Design review of the part built by this model. Coordinates are the model's own, in mm. A direction names the side the tool comes from. Give positions to 0.01 mm unless a question says otherwise; leave off trailing zeros. Write each loop counter-clockwise with the first axis right and the second up, starting at its lowest first coordinate (ties: lowest second). Pieces come first, ordered by that corner, then holes. Notation, with made-up numbers: (32.25, -19) -> (87.25, -19) arc R25 cw to (87.25, 17) -> close; hole circle Ø10 at (-10, -8). An arc over 180 degrees is marked (long way). Use CSV: the item, a comma, the result in double quotes.
```python
from build123d import *

# Parameters (mm, degrees)
SKETCH_1_R      = 7
SKETCH_1_R_2    = 6
EXTRUDE_1_DEPTH = 1
SKETCH_1_4_R    = 6
SKETCH_1_4_R_2  = 5
EXTRUDE_2_DEPTH = 1.5
SKETCH_1_5_R    = 5
SKETCH_1_5_R_2  = 4.25
EXTRUDE_3_DEPTH = 12
EXTRUDE_START   = 5
SKETCH_1_6_R    = 4.25
SKETCH_1_6_W    = 5.5
SKETCH_1_6_H    = 5.5
EXTRUDE_4_DEPTH = 7
SKETCH_1_7_R    = 7
SKETCH_1_7_R_2  = 6
SKETCH_1_7_R_3  = 5
SKETCH_1_7_R_4  = 4.25
SKETCH_1_7_W    = 5.5
SKETCH_1_7_H    = 5.5
SKETCH_1_7_R_5  = 2.1
EXTRUDE_5_DEPTH = 6
FILLET_1_R      = 1
CHAMFER_1_SIZE  = 0.2
CHAMFER_2_SIZE  = 0.3
CHAMFER_3_SIZE  = 0.3


with BuildPart() as part:
    # Sketch 1 → Extrude 1 (new body)
    with BuildSketch(Plane(origin=(0, 0, 0), x_dir=(1, 0, 0), z_dir=(0, 1, 0))):
        with Locations(Location((0, 0, 0), (0, 0, 270))):
            Circle(SKETCH_1_R)
        with Locations(Location((0, 0, 0), (0, 0, 270))):
            Circle(SKETCH_1_R_2, mode=Mode.SUBTRACT)
    extrude(amount=EXTRUDE_1_DEPTH)

    # Sketch 1_4 → Extrude 2 (add)
    with BuildSketch(Plane(origin=(0, 0, 0), x_dir=(1, 0, 0), z_dir=(0, 1, 0))):
        with Locations(Location((0, 0, 0), (0, 0, 270))):
            Circle(SKETCH_1_4_R)
        with Locations(Location((0, 0, 0), (0, 0, 270))):
            Circle(SKETCH_1_4_R_2, mode=Mode.SUBTRACT)
    extrude(amount=EXTRUDE_2_DEPTH)

    # Sketch 1_5 → Extrude 3 (add)
    with BuildSketch(Plane(origin=(0, 0, 0), x_dir=(1, 0, 0), z_dir=(0, 1, 0))):
        with Locations(Location((0, 0, 0), (0, 0, 270))):
            Circle(SKETCH_1_5_R)
        with Locations(Location((0, 0, 0), (0, 0, 270))):
            Circle(SKETCH_1_5_R_2, mode=Mode.SUBTRACT)
    extrude(amount=EXTRUDE_3_DEPTH)

    # Sketch 1_6 → Extrude 4 (add)
    with BuildSketch(Plane(origin=(0, 0, 0), x_dir=(1, 0, 0), z_dir=(0, 1, 0)).offset(EXTRUDE_START)):
        with Locations(Location((0, 0, 0), (0, 0, 270))):
            Circle(SKETCH_1_6_R)
        Rectangle(SKETCH_1_6_W, SKETCH_1_6_H, mode=Mode.SUBTRACT)
    extrude(amount=EXTRUDE_4_DEPTH)

    # Sketch 1_7 → Extrude 5 (add)
    # profile 1 of 3: a face of its own
    with BuildSketch(Plane(origin=(0, 0, 0), x_dir=(1, 0, 0), z_dir=(0, 1, 0)).offset(EXTRUDE_START)):
        with Locations(Location((0, 0, 0), (0, 0, 270))):
            Circle(SKETCH_1_7_R)
        with Locations(Location((0, 0, 0), (0, 0, 270))):
            Circle(SKETCH_1_7_R_2, mode=Mode.SUBTRACT)
    # profile 2 of 3: a face of its own
    with BuildSketch(Plane(origin=(0, 0, 0), x_dir=(1, 0, 0), z_dir=(0, 1, 0)).offset(EXTRUDE_START)):
        with Locations(Location((0, 0, 0), (0, 0, 270))):
            Circle(SKETCH_1_7_R_3)
        with Locations(Location((0, 0, 0), (0, 0, 270))):
            Circle(SKETCH_1_7_R_4, mode=Mode.SUBTRACT)
    # profile 3 of 3: a face of its own
    with BuildSketch(Plane(origin=(0, 0, 0), x_dir=(1, 0, 0), z_dir=(0, 1, 0)).offset(EXTRUDE_START)):
        Rectangle(SKETCH_1_7_W, SKETCH_1_7_H)
        with Locations(Location((0, 0, 0), (0, 0, 270))):
            Circle(SKETCH_1_7_R_5, mode=Mode.SUBTRACT)
    extrude(amount=EXTRUDE_5_DEPTH)


with BuildPart() as extrude_5_kept_piece:
    # of the separate pieces the step leaves, the one the design keeps (extrude_5_pieces_kept)
    add(part.part.solids().sort_by_distance((0, 0, 7))[0])

    # Fillet 1
    fillet_1_edges = [extrude_5_kept_piece.edges().sort_by_distance(p)[0] for p in [
        (2.75, 11.5, -2.75),
        (2.75, 11.5, 2.75),
        (-2.75, 11.5, 2.75),
        (-2.75, 11.5, -2.75),
    ]]
    fillet(fillet_1_edges, radius=FILLET_1_R)

    # Chamfer 1
    chamfer_1_edges = [extrude_5_kept_piece.edges().sort_by_distance(p)[0] for p in [
        (0, 1.5, -6),
        (0, 1, -7),
        (0, 12, -5),
        (0, 0, -7),
    ]]
    chamfer(chamfer_1_edges, length=CHAMFER_1_SIZE)

    # Chamfer 2
    chamfer_2_edges = [extrude_5_kept_piece.edges().sort_by_distance(p)[0] for p in [
        (0, 0, -4.25),
    ]]
    chamfer(chamfer_2_edges, length=CHAMFER_2_SIZE)

    # Chamfer 3
    chamfer_3_edges = [extrude_5_kept_piece.edges().sort_by_distance(p)[0] for p in [
        (0, 11, -2.1),
        (0, 12, 2.75),
        (2.75, 12, 0),
        (-2.75, 12, 0),
        (0, 12, -2.75),
        (2.457106781, 12, 2.457106781),
        (-2.457106781, 12, 2.457106781),
        (2.457106781, 12, -2.457106781),
        (-2.457106781, 12, -2.457106781),
    ]]
    chamfer(chamfer_3_edges, length=CHAMFER_3_SIZE)


solid = extrude_5_kept_piece.part
```
(1) For line 1 along X through (y, z) = (7.25, 0); line 2 along X through (y, z) = (4, 0); line 3 along Y through (x, z) = (2, -4.75), list the stretches that pass through material, from the lowest coordinate up. Write a range as [from, to].
Established:
line 1,"x = [-5, -2.1], [2.1, 5]"
line 2,"x = [-5, -4.25], [4.25, 5]"
line 3,"y = [0, 1.5]"
(2) Mouldability with a two-part tool opening along X and no side actions: class faces 4 (the face through (2.465, 11.355, 2.449)), 5 (the face through (-2.3, 1.15, 5.54)), 6 (the face through (2, 5, 2)) as +X half, -X half, draft (parallel to the pull), parting line (faces both ways), or undercut.
Established:
face 4,"undercut"
face 5,"parting line"
face 6,"undercut"
(3) Tool access review of faces 1 (the face through (4.214, 2.617, -0.553)), 2 (the face through (2.465, 11.355, -2.449)), 3 (the face through (0.631, 7.81, 2.003)): name each direction out of +Z, -Z, +X, -X, +Y, -Y from which nothing blocks a thin tool from reaching the whole face with its end or side.
Established:
face 1,"-Y"
face 2,"+Y"
face 3,"+Y, -Y"
(4) Take a section at A-A (y = 11.25). Write out the cut boundary in (x, z).
Established:
outline,"circle Ø10 at (0, 0); hole (-2.75, -1.75) arc R1 ccw to (-1.75, -2.75) -> (1.75, -2.75) arc R1 ccw to (2.75, -1.75) -> (2.75, 1.75) arc R1 ccw to (1.75, 2.75) -> (-1.75, 2.75) arc R1 ccw to (-2.75, 1.75) -> close"
(5) Take a section at B-B (y = 7.5). Write out the cut boundary in (x, z).
Established:
outline,"circle Ø10 at (0, 0); hole circle Ø4.2 at (0, 0)"
(6) Clearance check with flat-ended pins moving along their axes: pin 1 (4 mm diameter, centred on x = 1, z = 1.5, fed in from -Y); pin 2 (1.5 mm diameter, centred on x = 5, z = 5.5, fed in from +Y); pin 3 (0.6 mm diameter, centred on y = 11.5, z = -0.5, fed in from +X). State where each tip first meets the part, or that it passes through.
Established:
pin 1,"stops at y = 5"
pin 2,"stops at y = 1"
pin 3,"stops at x = 5"
